Can you work these out from the model? Positions are in its coordinate system, mm. A direction names the side the tool comes from. Give positions to 0.01 mm unless a question says otherwise; leave off trailing zeros. Loops run counter-clockwise (first coordinate to the right, second up) from the corner with the lowest first, then second, coordinate; pieces in that order, holes last. Notation, with made-up numbers: M -31.75,19 L -17.75,19 A36 ccw -17.75,55 Z; hole C 36.25,-21 d9. An arc over 180 degrees is marked long. Use CSV: the item, a comma, the result in double quotes.
from build123d import *

# Parameters (mm, degrees)
F0_R     = 7.5
F1_DEPTH = 3
F2_SIZE2 = 2.99999
F2_SIZE  = 1.99999
F3_R     = 2.4
F4_DEPTH = 5
F5_R     = 1


# Not quite as in the source:
# - a fillet or chamfer is up to 0.001 mm smaller than in the source, because OpenCascade refuses the exact size


with BuildPart() as f1:
    # F0 (on Top) → F1 (new body)
    with BuildSketch(Plane.XY):
        Circle(F0_R)
    extrude(amount=F1_DEPTH)

    # F2 (size 2 and 3 in the source; OpenCascade refuses exactly that, so slightly less here)
    f2_edges = [f1.edges().sort_by_distance(p)[0] for p in [
        (-7.5, 0, 3),
    ]]
    f2_side = f1.faces().sort_by_distance((0, 0, 3))[0]
    chamfer(f2_edges, length=F2_SIZE, length2=F2_SIZE2, reference=f2_side)

    # F3 (on face) → F4 (join)
    with BuildSketch(Plane.XY.offset(3)):
        Circle(F3_R)
    extrude(amount=F4_DEPTH)

    # F5
    f5_edges = [f1.edges().sort_by_distance(p)[0] for p in [
        (-2.4, 0, 8),
        (-2.4, 0, 3),
    ]]
    fillet(f5_edges, radius=F5_R)

    # F6 (on Right) → F7 (revolve, cut)
    with BuildSketch(Plane.YZ):
        with BuildLine():
            Line((0, 0), (0, 1))
            ThreePointArc((0, 1), (-18.0312229203, -6.4687770797), (-25.5, -24.5))
            Line((-25.5, -24.5), (0, -24.5))
            Line((0, -24.5), (0, 0))
        make_face()
    revolve(axis=Axis((0, 0, -12.25), (0, 0, -1)), mode=Mode.SUBTRACT)


solid = f1.part
Q1. For faces 1 (the cylindrical face through (1.29, 2.024, 5.479)), 2 (the flat face through (-7, 2, 0)), which set-ups out of +Z, -Z, +X, -X, +Y, -Y let a thin tool reach every point of the face, with its end or its side?
Model answer:
face 1,"+Z"
face 2,"-Z, +X, -X, +Y, -Y"
Q2. I want a section at C-C, the plane z = 2.25. Please give me the cut outline in (x, y).
Model answer:
outline,"C 0,0 d12"
Q3. I'm going to push flat-ended pins straight in: P1, Ø1, axis at y = -1.5, z = 5, coming from the +X side; P2, Ø1.5, axis at x = 1.5, z = 5, coming from the +Y side; P3, Ø2, axis at x = -2, y = -5.5, coming from the -Z side. Where does each tip first touch, or does it pass through?
Model answer:
P1,"x = 2.18"
P2,"y = 2.28"
P3,"z = 0.06"
Q4. Please list where these lines run through material, in increasing order: L1, parallel to X at y = 1.5, z = 4.25; L2, parallel to Y at x = 0, z = 1.25; L3, parallel to Y at x = 0.75, z = 2. Write a range as from..to.
Model answer:
L1,"-1.87..1.87"
L2,"-6.67..6.67"
L3,"-6.12..6.12"
Q5. I want a section at D-D, the plane z = 6.75. Please give me the cut outline in (x, y), then the cut area to 3 significant figures.
Model answer:
outline,"C 0,0 d4.8"
area,"18.1 mm2"
